The model under review builds one solid part; all positions refer to its coordinate system, in mm. Face numbers are marked on the shaded views. A direction names the side the tool comes from. Coordinates: 2 decimals unless noted, no trailing zeros. Loops run counter-clockwise (first coordinate to the right, second up) from the corner with the lowest first, then second, coordinate; pieces in that order, holes last. Notation, with made-up numbers: (-2.75, -4.75) - (34.25, -4.75) arc R28 cw to (34.25, 20.25) - close; hole circle Ø2 at (-16.75, -26.5). An arc over 180 degrees is marked (long way). Answer in a Markdown table with one row per item. Add a question column.
(1) For line 1 along X through (y, z) = (2.5, -0.75); line 2 along Y through (x, z) = (0, 12.6), list the stretches that pass through material, from the lowest coordinate up.
(2) We need section A-A on z = 0. Write out the cut boundary in (x, y), plus the area to 3 significant figures.
(3) We need section C-C on y = 1.5. Write out the cut boundary in (x, z).
(4) We need section B-B on x = 4.75. Write out the cut boundary in (y, z), plus the area to 3 significant figures.
(5) We need section D-D on x = 0. Write out the cut boundary in (y, z).
(6) Mouldability with a two-part tool opening along X and no side actions: class the marked faces 1, 2 and 3 as +X half, -X half, draft (parallel to the pull), parting line (faces both ways), or undercut.
(7) Machinability: for the marked faces 4 and 5, which of the approach directions +Z, -Z, +X, -X, +Y, -Y give a long, thin tool a straight path to every point of the face, cutting with its end or side? Answer none if there is none.
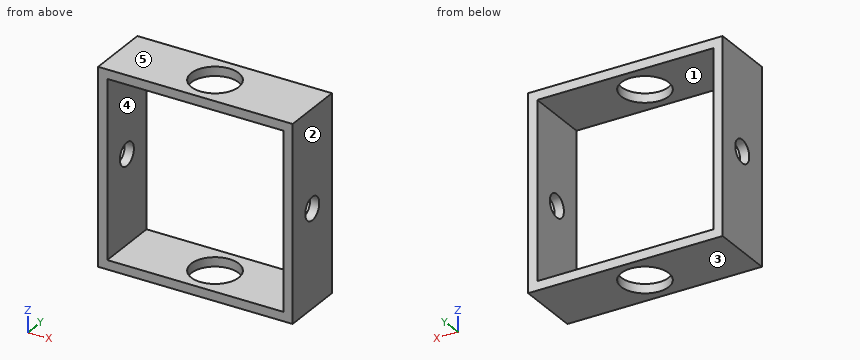
from build123d import *

# Parameters (mm, degrees)
SKETCH1_W           = 26.9875
SKETCH1_H           = 26.9875
SKETCH1_W_2         = 24.4475
SKETCH1_H_2         = 24.4475
BOSS_EXTRUDE1_DEPTH = 8.89
SKETCH2_R           = 1.5875
CUT_EXTRUDE1_DEPTH  = 152.4
SKETCH3_R           = 3.302
CUT_EXTRUDE3_DEPTH  = 152.4


with BuildPart() as part:
    # Sketch1 → Boss-Extrude1 (new body)
    with BuildSketch(Plane(origin=(0, 0, 0), x_dir=(1, 0, 0), z_dir=(0, 1, 0))):
        Rectangle(SKETCH1_W, SKETCH1_H)
        Rectangle(SKETCH1_W_2, SKETCH1_H_2, mode=Mode.SUBTRACT)
    extrude(amount=BOSS_EXTRUDE1_DEPTH)

    # Sketch2 → Cut-Extrude1 (cut)
    with BuildSketch(Plane(origin=(13.49375, 0, 0), x_dir=(0, 0, -1), z_dir=(1, 0, 0))):
        with Locations((0, 4.445)):
            Circle(SKETCH2_R)
    extrude(amount=-CUT_EXTRUDE1_DEPTH, mode=Mode.SUBTRACT)

    # Sketch3 → Cut-Extrude3 (cut)
    with BuildSketch(Plane(origin=(0, 0, -13.49375), x_dir=(-1, 0, 0), z_dir=(0, 0, -1))):
        with Locations((0, 4.445)):
            Circle(SKETCH3_R)
    extrude(amount=-CUT_EXTRUDE3_DEPTH, mode=Mode.SUBTRACT)


solid = part.part
Outcome:
| question | item | result |
|---|---|---|
| 1 | line 1 | -13.49 to -12.22, 12.22 to 13.49 |
| 1 | line 2 | 0 to 1.14, 7.75 to 8.89 |
| 2 | outline | (-13.49, 0) - (-12.22, 0) - (-12.22, 2.86) - (-13.49, 2.86) - close; (-13.49, 6.03) - (-12.22, 6.03) - (-12.22, 8.89) - (-13.49, 8.89) - close; (12.22, 0) - (13.49, 0) - (13.49, 2.86) - (12.22, 2.86) - close; (12.22, 6.03) - (13.49, 6.03) - (13.49, 8.89) - (12.22, 8.89) - close |
| 2 | area | 14.5 mm² |
| 3 | outline | (-13.49, -13.49) - (-1.49, -13.49) - (-1.49, -12.22) - (-12.22, -12.22) - (-12.22, 12.22) - (-1.49, 12.22) - (-1.49, 13.49) - (-13.49, 13.49) - close; (1.49, -13.49) - (13.49, -13.49) - (13.49, 13.49) - (1.49, 13.49) - (1.49, 12.22) - (12.22, 12.22) - (12.22, -12.22) - (1.49, -12.22) - close |
| 4 | outline | (0, -13.49) - (8.89, -13.49) - (8.89, -12.22) - (0, -12.22) - close; (0, 12.22) - (8.89, 12.22) - (8.89, 13.49) - (0, 13.49) - close |
| 4 | area | 22.6 mm² |
| 5 | outline | (0, -13.49) - (1.14, -13.49) - (1.14, -12.22) - (0, -12.22) - close; (0, 12.22) - (1.14, 12.22) - (1.14, 13.49) - (0, 13.49) - close; (7.75, -13.49) - (8.89, -13.49) - (8.89, -12.22) - (7.75, -12.22) - close; (7.75, 12.22) - (8.89, 12.22) - (8.89, 13.49) - (7.75, 13.49) - close |
| 6 | face 1 | undercut |
| 6 | face 2 | +X half |
| 6 | face 3 | draft |
| 7 | face 4 | +Y, -Y |
| 7 | face 5 | +Z, +X, -X, +Y, -Y |
